For this review, take the finished solid that the model builds, in its own axes (mm). A direction names the side the tool comes from. Round coordinates to 2 decimals unless told otherwise and drop trailing zeros. Loops run counter-clockwise (first coordinate to the right, second up) from the corner with the lowest first, then second, coordinate; pieces in that order, holes last.
1. Tool access review of faces 4 (the cylindrical face through (-98.93, 8.98, -29.41)), 5 (the cylindrical face through (-33.202, -0.507, -24.985)), 6 (the cylindrical face through (-32.594, 10.452, -26.82)): name each direction out of +Z, -Z, +X, -X, +Y, -Y from which nothing blocks a thin tool from reaching the whole face with its end or side.
2. Consider section A-A on y = 4. State the section outline as (x, z) points (3 decimals), then the cut area to 3 significant figures.
3. Consider section D-D on y = 12. State the section outline as (x, z) points (3 decimals).
4. Consider section C-C on z = -13.5. State the section outline as (x, y) points.
5. Clearance check with flat-ended pins moving along their axes: pin 1 Ø17.5 at (x, z) = (-65.5, -5.5) entering from -Y; pin 2 Ø4 at (x, z) = (-105.93, -27.14) entering from -Y; pin 3 Ø0.5 at (x, y) = (-80, -0.5) entering from -Z. State where each tip first meets the part, or that it passes through.
6. Draft analysis for pull direction Y (two halves, no side actions). For faces 1 (the flat face through (-30.63, 9, -2)), 2 (the flat face through (-68, 20, -2)), 3 (the cylindrical face through (-98.93, 3.98, -29.41)), state which applies: released by +Y, released by -Y, zero draft, split by the parting line, or undercut.
7. Consider section B-B on x = -75.5. State the section outline as (y, z) points, then the cut area to 3 significant figures.
8. To check wall thickness, follow line 1 along Z through (x, y) = (-56, 10.75); line 2 along X through (y, z) = (5.25, 10); line 3 along Y through (x, z) = (-51, -9.5). State the ranges of each line that lie inside material, in increasing order.
from build123d import *

# Parameters (mm, degrees)
SKETCH1_W           = 82.8
SKETCH1_H           = 57.7
BOSS_EXTRUDE1_DEPTH = 21.2
SKETCH2_R           = 1.5
CUT_EXTRUDE1_DEPTH  = 22
CUT_EXTRUDE2_DEPTH  = 20
FILLET3_R           = 4
BOSS_EXTRUDE3_START = 1
BOSS_EXTRUDE3_DEPTH = 1
CUT_EXTRUDE6_DEPTH  = 126.949440358
SKETCH8_R           = 3.8
CUT_EXTRUDE7_DEPTH  = 91.96532852


with BuildPart() as part:
    # Sketch1 → Boss-Extrude1 (new body)
    with BuildSketch(Plane(origin=(0, 0, 0), x_dir=(1, 0, 0), z_dir=(0, 1, 0))):
        with Locations((-68.529666271, 2.285365627)):
            Rectangle(SKETCH1_W, SKETCH1_H)
    extrude(amount=BOSS_EXTRUDE1_DEPTH)

    # Sketch2 → Cut-Extrude1 (cut)
    with BuildSketch(Plane.XZ):
        with Locations(Location((-105.929666271, 22.574078856, 0), (0, 0, 270))):
            Circle(SKETCH2_R)
        with Locations(Location((-31.129666271, 22.574078856, 0), (0, 0, 270))):
            Circle(SKETCH2_R)
        with Locations(Location((-105.929666271, -27.14481011, 0), (0, 0, 270))):
            Circle(SKETCH2_R)
        with Locations(Location((-31.129666271, -27.14481011, 0), (0, 0, 270))):
            Circle(SKETCH2_R)
    extrude(amount=-CUT_EXTRUDE1_DEPTH, mode=Mode.SUBTRACT)

    # Sketch3 → Cut-Extrude2 (cut)
    with BuildSketch(Plane.XZ):
        with BuildLine():
            Line((-101.969305307, 23.064634373), (-35.090027235, 23.064634373))
            ThreePointArc((-35.090027235, 23.064634373), (-33.948648913, 19.745651731), (-30.629666271, 18.604273409))
            Line((-30.629666271, 18.604273409), (-30.629666271, -23.175004663))
            ThreePointArc((-30.629666271, -23.175004663), (-33.948648913, -24.316382985), (-35.090027235, -27.635365627))
            Line((-35.090027235, -27.635365627), (-101.969305307, -27.635365627))
            ThreePointArc((-101.969305307, -27.635365627), (-103.110683629, -24.316382985), (-106.429666271, -23.175004663))
            Line((-106.429666271, -23.175004663), (-106.429666271, 18.607164142))
            ThreePointArc((-106.429666271, 18.607164142), (-103.111962249, 19.747670443), (-101.969305307, 23.064634373))
        make_face()
    extrude(amount=-CUT_EXTRUDE2_DEPTH, mode=Mode.SUBTRACT)

    # Fillet3
    fillet3_edges = [part.edges().sort_by_distance(p)[0] for p in [
        (-27.129666271, 10.6, 26.564634373),
        (-109.929666271, 10.6, 26.564634373),
        (-109.929666271, 10.6, -31.135365627),
        (-27.129666271, 10.6, -31.135365627),
    ]]
    fillet(fillet3_edges, radius=FILLET3_R)

    # Sketch3_8 → Boss-Extrude3 (add)
    with BuildSketch(Plane.XZ.offset(BOSS_EXTRUDE3_START)):
        with BuildLine():
            Line((-103.334287863, 24.064634373), (-33.723727934, 24.064634373))
            ThreePointArc((-33.723727934, 24.064634373), (-33.241542132, 20.452758513), (-29.629666271, 19.97057271))
            Line((-29.629666271, 19.97057271), (-29.629666271, -24.541303964))
            ThreePointArc((-29.629666271, -24.541303964), (-33.241542132, -25.023489766), (-33.723727934, -28.635365627))
            Line((-33.723727934, -28.635365627), (-103.335604608, -28.635365627))
            ThreePointArc((-103.335604608, -28.635365627), (-103.817790411, -25.023489766), (-107.429666271, -24.541303964))
            Line((-107.429666271, -24.541303964), (-107.429666271, 19.973301106))
            ThreePointArc((-107.429666271, 19.973301106), (-103.819200468, 20.454646008), (-103.334287863, 24.064634373))
        make_face()
        with BuildLine():
            Line((-101.969305307, 23.064634373), (-35.090027235, 23.064634373))
            ThreePointArc((-35.090027235, 23.064634373), (-33.948648913, 19.745651731), (-30.629666271, 18.604273409))
            Line((-30.629666271, 18.604273409), (-30.629666271, -23.175004663))
            ThreePointArc((-30.629666271, -23.175004663), (-33.948648913, -24.316382985), (-35.090027235, -27.635365627))
            Line((-35.090027235, -27.635365627), (-101.969305307, -27.635365627))
            ThreePointArc((-101.969305307, -27.635365627), (-103.110683629, -24.316382985), (-106.429666271, -23.175004663))
            Line((-106.429666271, -23.175004663), (-106.429666271, 18.607164142))
            ThreePointArc((-106.429666271, 18.607164142), (-103.111962249, 19.747670443), (-101.969305307, 23.064634373))
        make_face(mode=Mode.SUBTRACT)
    extrude(amount=-BOSS_EXTRUDE3_DEPTH)

    # Sketch7 → Cut-Extrude6 (cut, through all)
    with BuildSketch(Plane(origin=(0, 0, -31.135365627), x_dir=(-1, 0, 0), z_dir=(0, 0, -1))):
        with BuildLine():
            Line((97.929666271, 10), (60.929666271, 10))
            ThreePointArc((60.929666271, 10), (59.929666271, 9), (60.929666271, 8))
            Line((60.929666271, 8), (97.929666271, 8))
            ThreePointArc((97.929666271, 8), (98.929666271, 9), (97.929666271, 10))
        make_face()
        with BuildLine():
            Line((97.929666271, 5), (60.929666271, 5))
            ThreePointArc((60.929666271, 5), (59.929666271, 4), (60.929666271, 3))
            Line((60.929666271, 3), (97.929666271, 3))
            ThreePointArc((97.929666271, 3), (98.929666271, 4), (97.929666271, 5))
        make_face()
    extrude(amount=-CUT_EXTRUDE6_DEPTH, mode=Mode.SUBTRACT)

    # Sketch8 → Cut-Extrude7 (cut, through all)
    with BuildSketch(Plane.ZY.offset(109.929666271)):
        with Locations((14.564634373, 9.2)):
            Circle(SKETCH8_R)
    extrude(amount=-CUT_EXTRUDE7_DEPTH, mode=Mode.SUBTRACT)


solid = part.part
Resolved:
1. face 4: +Z, -Z
1. face 5: -Y
1. face 6: +Y, -Y
2. outline: (-109.93, -27.135) arc R4 ccw to (-105.93, -31.135) - (-98.93, -31.135) - (-98.93, -27.635) - (-101.969, -27.635) arc R4 ccw to (-106.43, -23.175) - (-106.43, 18.607) arc R4 ccw to (-101.969, 23.065) - (-98.93, 23.065) - (-98.93, 26.565) - (-105.93, 26.565) arc R4 ccw to (-109.93, 22.565) - close; (-59.93, -31.135) - (-31.13, -31.135) arc R4 ccw to (-27.13, -27.135) - (-27.13, 22.565) arc R4 ccw to (-31.13, 26.565) - (-59.93, 26.565) - (-59.93, 23.065) - (-35.09, 23.065) arc R4 ccw to (-30.63, 18.604) - (-30.63, -23.175) arc R4 ccw to (-35.09, -27.635) - (-59.93, -27.635) - close; hole circle Ø3 at (-105.93, -27.145); hole circle Ø3 at (-105.93, 22.574); hole circle Ø3 at (-31.13, -27.145); hole circle Ø3 at (-31.13, 22.574)
2. area: 686 mm2
3. outline: (-109.93, -27.135) arc R4 ccw to (-105.93, -31.135) - (-31.13, -31.135) arc R4 ccw to (-27.13, -27.135) - (-27.13, 11.996) - (-30.63, 11.996) - (-30.63, -23.175) arc R4 ccw to (-35.09, -27.635) - (-101.969, -27.635) arc R4 ccw to (-106.43, -23.175) - (-106.43, 11.996) - (-109.93, 11.996) - close; (-109.93, 17.134) - (-106.43, 17.134) - (-106.43, 18.607) arc R4 ccw to (-101.969, 23.065) - (-35.09, 23.065) arc R4 ccw to (-30.63, 18.604) - (-30.63, 17.134) - (-27.13, 17.134) - (-27.13, 22.565) arc R4 ccw to (-31.13, 26.565) - (-105.93, 26.565) arc R4 ccw to (-109.93, 22.565) - close; hole circle Ø3 at (-105.93, -27.145); hole circle Ø3 at (-105.93, 22.574); hole circle Ø3 at (-31.13, -27.145); hole circle Ø3 at (-31.13, 22.574)
4. outline: (-109.93, 0) - (-107.43, 0) - (-107.43, -1) - (-106.43, -1) - (-106.43, 20) - (-30.63, 20) - (-30.63, -1) - (-29.63, -1) - (-29.63, 0) - (-27.13, 0) - (-27.13, 21.2) - (-109.93, 21.2) - close
5. pin 1: stops at y = 20
5. pin 2: stops at y = 0
5. pin 3: stops at z = -28.64
6. face 1: zero draft
6. face 2: released by -Y
6. face 3: undercut
7. outline: (-1, -28.64) - (0, -28.64) - (0, -31.14) - (3, -31.14) - (3, -27.64) - (-1, -27.64) - close; (-1, 23.06) - (3, 23.06) - (3, 26.56) - (0, 26.56) - (0, 24.06) - (-1, 24.06) - close; (5, -31.14) - (8, -31.14) - (8, -27.64) - (5, -27.64) - close; (5, 23.06) - (8, 23.06) - (8, 26.56) - (5, 26.56) - close; (10, -31.14) - (21.2, -31.14) - (21.2, 26.56) - (10, 26.56) - (10, 23.06) - (20, 23.06) - (20, -27.64) - (10, -27.64) - close
7. area: 183 mm2
8. line 1: z = -31.14 to -27.64, 23.06 to 26.56
8. line 2: x = -109.93 to -106.43, -30.63 to -27.13
8. line 3: y = 20 to 21.2
